Autodesk Inventor part; units mm, degrees
ref_plane "YZ Plane" through (0, 0, 0) normal (1, 0, 0) x (0, 1, 0)
ref_plane "XZ Plane" through (0, 0, 0) normal (0, 1, 0) x (-1, 0, 0)
ref_plane "XY Plane" through (0, 0, 0) normal (0, 0, 1) x (1, 0, 0)
sketch "Эскиз1" plane through (0, 0, 0) normal (0, 0, 1) x (1, 0, 0)
  line L0 (0, 0) -> (-11.15, 0)
  line L1 (-11.15, 0) -> (-9.75, 67.9856)
  line L2 (-9.75, 67.9856) -> (0, 67.9856)
  line L3 (0, 67.9856) -> (0, 0)
  line L4 (0, 67.9856) -> (0, 70.4856)
  line L5 (-9.75, 67.9856) -> (-9.6985, 70.4856)
  line L6 (0, 70.4856) -> (-9.6985, 70.4856)
  dimension "d0" = 11.15
  dimension "d1" = 9.75
  dimension "d2" = 68
  dimension "d3" = 2.5
revolve "Вращение1" add sketch "Эскиз1" angle 360 about axis through (0, 67.9856, 0) along (0, -1, 0)
fillet "Сопряжение1" radius 2 1 edges at (9.6985, 70.4856, 0)
sketch "Эскиз2" plane through (0, 0, 0) normal (0, 0, 1) x (1, 0, 0)
  line L0 (-7.7393, 70.4856) -> (7.7393, 70.4856)
  line L1 (0, 70.4856) -> (0, 72.9856)
  line L2 (0, 72.9856) -> (-7.2, 72.9856)
  line L3 (-7.2, 72.9856) -> (-7.7, 70.4856)
  line L4 (0, 72.9856) -> (-7.2, 72.9856)
  line L5 (-7.2, 72.9856) -> (-7.2, 74.9856)
  line L6 (-7.2, 74.9856) -> (0, 74.9856)
  line L7 (0, 74.9856) -> (0, 72.9856)
  line L8 (-7.2, 75.9856) -> (0, 75.9856)
  line L9 (0, 75.9856) -> (0, 74.9856)
  arc A0 (-7.2, 75.9856) -> (-7.2, 74.9856) centre (-4.725, 75.4856) ccw
  line L10 (-7.2, 75.9856) -> (-4.3, 79.9856)
  line L11 (-4.3, 79.9856) -> (0, 79.9856)
  line L12 (0, 79.9856) -> (0, 75.9856)
  line L13 (-4.3, 79.9856) -> (0, 79.9856)
  line L14 (0, 79.9856) -> (0, 87.4856)
  line L15 (0, 87.4856) -> (-4.3, 87.4856)
  line L16 (-4.3, 87.4856) -> (-4.3, 79.9856)
  arc A1 (-5.025, 78.9856) -> (-4.3, 81.2207) centre (-8.108, 81.2207) ccw
  line L17 (0, 87.4856) -> (-3.075, 87.4856)
  line L18 (-3.075, 87.4856) -> (-3.075, 90.9856)
  line L19 (-3.075, 90.9856) -> (0, 90.9856)
  line L20 (0, 90.9856) -> (0, 87.4856)
  line L21 (-3.075, 90.9856) -> (-1.5669, 95.3677)
  arc A2 (0, 96.4856) -> (-1.5669, 95.3677) centre (0, 94.8285) ccw
  line L22 (0, 90.9856) -> (0, 96.4856)
  point P0 (0, 0)
  point P1 (-7.25, 75.4856)
  point P2 (-3.075, 87.4856)
  dimension "d6" = 7.2
  dimension "d7" = 7.7
  dimension "d8" = 2.5
  dimension "d9" = 2
  dimension "d10" = 1
  dimension "d12" = 0.05
  dimension "d13" = 4.3
  dimension "d14" = 4
  dimension "d15" = 17
  dimension "d16" = 1
  dimension "d17" = 1.2352
  dimension "d18" = 3.075
  dimension "d19" = 3.5
  dimension "d20" = 5.5
revolve "Вращение2" add sketch "Эскиз2" angle 360 about axis through (0, 79.9856, 0) along (0, 1, 0)
sketch "Эскиз3" plane through (0, 0, 0) normal (0, -1, 0) x (1, 0, 0)
  circle A0 centre (0, 0) radius 11.15
extrude "Выдавливание1" add sketch "Эскиз3" along normal blind 1.5
sketch "Эскиз4" plane through (0, 0, 0) normal (0, 0, 1) x (1, 0, 0)
  line L0 (-11.15, -1.5) -> (11.15, -1.5)
  line L1 (0, -1.5) -> (0, -24)
  line L2 (0, -24) -> (-9.6, -24)
  line L3 (-9.6, -24) -> (-9.75, -1.5)
  line L4 (-9.75, -1.5) -> (0, -1.5)
  line L5 (-9.6, -24) -> (-9.5833, -26.5)
  line L6 (-9.5833, -26.5) -> (0, -26.5)
  line L7 (0, -26.5) -> (0, -24)
  arc A0 (-9.6, -24) -> (-9.2661, -26.5) centre (0.4274, -23.9332) ccw
  line L8 (0, -26.5) -> (-7.4, -26.5)
  line L9 (-7.4, -26.5) -> (-7.4, -29)
  line L10 (-7.4, -29) -> (0, -29)
  line L11 (0, -29) -> (0, -26.5)
  line L12 (0, -29) -> (-7.2, -29)
  line L13 (-7.2, -29) -> (-7.2, -31.5)
  line L14 (-7.2, -31.5) -> (0, -31.5)
  line L15 (0, -31.5) -> (0, -29)
  line L16 (-7.2, -31.5) -> (0, -33)
  line L17 (0, -31.5) -> (0, -33)
  point P0 (0, 0)
  point P1 (-9.75, -1.5)
  dimension "d24" = 9.6
  dimension "d25" = 9.75
  dimension "d26" = 22.5
  dimension "d27" = 2.5
  dimension "d28" = 2.5
  dimension "d29" = 7.4
  dimension "d30" = 2.5
  dimension "d31" = 7.2
  dimension "d32" = 1.5
revolve "Вращение3" add sketch "Эскиз4" angle 360 about axis through (0, -29, 0) along (0, 1, 0) contours L0 L1 L2 L3 | L2 L7 L6 A0 | L11 L10 L9 L6 | L15 L14 L13 L10 | L17 L16 L14
sketch "Эскиз5" plane through (0, -1.5, 0) normal (0, -1, 0) x (1, 0, 0)
  circle A0 centre (0, 0) radius 11.15
  circle A1 centre (9.346, 0) radius 3
  circle A2 centre (0, 0) radius 11.15
  point P0 (0, 0)
  point P1 (10.8426, -2.6)
  point P2 (10.8426, 2.6)
  point P3 (10.8426, -2.6)
  dimension "d48" = 5.2
  dimension "d50" = 6
  dimension "d51" = 2.6
sketch "Эскиз6" plane through (0, -1.5, 0) normal (0, -1, 0) x (1, 0, 0)
  line L0 (10.35, 1.45) -> (8.1099, 1.45)
  line L1 (8.1099, 1.45) -> (8.1099, -1.45)
  line L2 (8.1099, -1.45) -> (10.35, -1.45)
  line L3 (10.35, -1.45) -> (10.35, 1.45)
  circle A0 centre (0, 0) radius 9.75
  point P0 (0, 0)
  dimension "d37" = 2.9
  dimension "d38" = 1.45
  dimension "d39" = 0.6
extrude "Выдавливание3" add sketch "Эскиз6" along normal blind 22.5 contours L3 L2 A0 L0 | A0 L2 L1 L0 picked at (8.6566, 0)
chamfer "Фаска1" distance 0.6 distance2 1.6 1 edges at (10.35, -24, 0) measured on face at (10.0959, -24, 0.1617)
pattern_circular "Круговой массив1" count 4 over 360 about axis through (0, -10, 0) along (0, 1, 0) of "Выдавливание3", "Фаска1"
extrude "Выдавливание4" add sketch "Эскиз5" against normal blind 1.5 contours A0 A1 picked at (11.5153, -0.4994)
properties part number "маркер"
Geometry: final body of the model. Coordinates: model frame, mm. A direction names the side the tool comes from. Give positions to 0.01 mm unless a question says otherwise; leave off trailing zeros. Order: outer loops, then holes, each group sorted by start corner. A loop starts at its lowest first (then second) coordinate and runs counter-clockwise, first axis right, second up. Notation, with made-up numbers: (21, 42.25) - (55, 42.25) arc R21 ccw to (55, 68.25) - close; hole circle Ø5 at (59, 13.25). An arc over 180 degrees is marked (long way). Use CSV: the item, a comma, the result in double quotes.
1. Access query for faces 1 (the face through (-6.781, -12.592, -6.903)), 2 (the face through (-2, 87.486, -3)), 3 (the face through (-6.87, -30.27, -2.16)). Directions: +Z, -Z, +X, -X, +Y, -Y. A direction counts if a zero-diameter tool reaches every point of the face in a straight line with its end or side. Return the directions, or none.
Answers below:
face 1,"-Z, -X, -Y"
face 2,"+Y"
face 3,"-Y"
2. Contact query for flat-ended pins moving along their axis: pin 1 (1 mm diameter, centred on x = -8, y = 31.5, fed in from +Z); pin 2 (2.5 mm diameter, centred on x = 0, y = -14.5, fed in from +Z); pin 3 (8 mm diameter, centred on y = -14.5, z = -2, fed in from -X). Output: stop coordinate, or through.
Answers below:
pin 1,"z = 7.35"
pin 2,"z = 10.35"
pin 3,"x = -10.35"
3. Section query A-A (y = 85). Output: boundary loops of the cut face in (x, z), plus the area to 3 significant figures.
Answers below:
outline,"circle Ø8.6 at (0, 0)"
area,"58.1 mm2"
4. Material intervals for line 1 along X through (y, z) = (66, 1); line 2 along X through (y, z) = (16.5, -8); line 3 along Z through (x, y) = (-7.75, 64), sorted ascending. Write a range as from..to.
Answers below:
line 1,"-9.74..9.74"
line 2,"-7.27..7.27"
line 3,"-6.05..6.05"
